Work out the finished part from the listing and answer in its coordinate system (mm). Face numbers are marked on the shaded views. A direction names the side the tool comes from. Coordinates: 2 decimals unless noted, no trailing zeros. Order: outer loops, then holes, each group sorted by start corner. A loop starts at its lowest first (then second) coordinate and runs counter-clockwise, first axis right, second up.
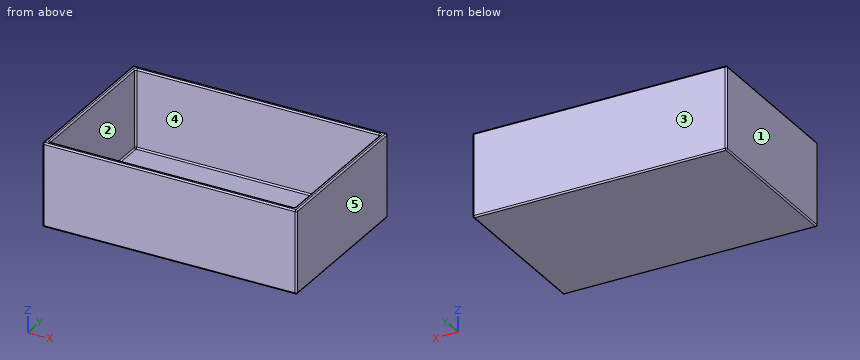
```python
from build123d import *

# Parameters (mm, degrees)
F0_W     = 524.05
F0_H     = 334.05
F0_W_2   = 505
F0_H_2   = 315
F1_DEPTH = 172.025
F2_DEPTH = 9.525
F3_R     = 3


with BuildPart() as f1:
    # F0 (on Top) → F1 (new body)
    with BuildSketch(Plane.XY):
        with Locations((48.210962, 70.14254)):
            Rectangle(F0_W, F0_H)
        with Locations((48.210962, 70.14254)):
            Rectangle(F0_W_2, F0_H_2, mode=Mode.SUBTRACT)
    extrude(amount=F1_DEPTH)

    # F0 (on Top) → F2 (join)
    with BuildSketch(Plane.XY):
        with Locations((48.210962, 70.14254)):
            Rectangle(F0_W_2, F0_H_2)
    extrude(amount=F2_DEPTH)

    # F3
    f3_edges = [f1.edges().sort_by_distance(p)[0] for p in [
        (-213.814038, -96.88246, 86.0125),
        (310.235962, -96.88246, 86.0125),
        (48.210962, -96.88246, 0),
        (48.210962, -96.88246, 172.025),
        (310.235962, 237.16754, 86.0125),
        (310.235962, 70.14254, 0),
        (310.235962, 70.14254, 172.025),
        (-213.814038, 237.16754, 86.0125),
        (48.210962, 237.16754, 0),
        (48.210962, 237.16754, 172.025),
        (-213.814038, 70.14254, 0),
        (-213.814038, 70.14254, 172.025),
        (300.710962, 70.14254, 172.025),
        (48.210962, -87.35746, 172.025),
        (-204.289038, 70.14254, 172.025),
        (48.210962, 227.64254, 172.025),
        (-204.289038, 70.14254, 9.525),
        (-204.289038, 227.64254, 90.775),
        (-204.289038, -87.35746, 90.775),
        (48.210962, -87.35746, 9.525),
        (300.710962, -87.35746, 90.775),
        (300.710962, 70.14254, 9.525),
        (300.710962, 227.64254, 90.775),
        (48.210962, 227.64254, 9.525),
    ]]
    fillet(f3_edges, radius=F3_R)


solid = f1.part
```
1. The part is cut by section C-C (x = -86.5). Determine the outline of the cut face in (y, z) (3 decimals), plus the area to 3 significant figures.
2. The part is cut by section A-A (z = 53.5). Determine the outline of the cut face in (x, y), plus the area to 3 significant figures.
3. For the marked faces 4 and 5, determine the directions among +Z, -Z, +X, -X, +Y, -Y from which every point of the face is accessible in a straight line to the end or side of a thin tool.
4. The part is cut by section B-B (y = 40). Determine the outline of the cut face in (x, z) (3 decimals).
5. The mould has two halves that part along Y. Classify the marked faces 1, 2 and 3: released by +Y, released by -Y, zero draft, split by the parting line, or undercut.
6. A flat-ended cylindrical pin translates along its axis: pin 1 (5 mm diameter, centred on x = -62.5, y = 81, fed in from +Z) (3 decimals). Find the tip coordinate at first contact, or state that the pin passes through.
7. Consider probe 1 along X at (y, z) = (198, 75); probe 2 along Y at (x, z) = (-106, 91); probe 3 along Z at (x, y) = (286.5, 118) (3 decimals). Determine where each line is inside the solid, lowest interval first.
Worked out:
1. outline: (-96.882, 3) arc R3 ccw to (-93.882, 0) - (234.168, 0) arc R3 ccw to (237.168, 3) - (237.168, 169.025) arc R3 ccw to (234.168, 172.025) - (230.643, 172.025) arc R3 ccw to (227.643, 169.025) - (227.643, 12.525) arc R3 cw to (224.643, 9.525) - (-84.357, 9.525) arc R3 cw to (-87.357, 12.525) - (-87.357, 169.025) arc R3 ccw to (-90.357, 172.025) - (-93.882, 172.025) arc R3 ccw to (-96.882, 169.025) - close
1. area: 6,270 mm2
2. outline: (-213.81, -93.88) arc R3 ccw to (-210.81, -96.88) - (307.24, -96.88) arc R3 ccw to (310.24, -93.88) - (310.24, 234.17) arc R3 ccw to (307.24, 237.17) - (-210.81, 237.17) arc R3 ccw to (-213.81, 234.17) - close; hole (-204.29, -84.36) arc R3 ccw to (-201.29, -87.36) - (297.71, -87.36) arc R3 ccw to (300.71, -84.36) - (300.71, 224.64) arc R3 ccw to (297.71, 227.64) - (-201.29, 227.64) arc R3 ccw to (-204.29, 224.64) - close
2. area: 16,000 mm2
3. face 4: +Z
3. face 5: +Z, -Z, +X, +Y, -Y
4. outline: (-213.814, 3) arc R3 ccw to (-210.814, 0) - (307.236, 0) arc R3 ccw to (310.236, 3) - (310.236, 169.025) arc R3 ccw to (307.236, 172.025) - (303.711, 172.025) arc R3 ccw to (300.711, 169.025) - (300.711, 12.525) arc R3 cw to (297.711, 9.525) - (-201.289, 9.525) arc R3 cw to (-204.289, 12.525) - (-204.289, 169.025) arc R3 ccw to (-207.289, 172.025) - (-210.814, 172.025) arc R3 ccw to (-213.814, 169.025) - close
5. face 1: zero draft
5. face 2: undercut
5. face 3: released by +Y
6. pin 1: stops at z = 9.525
7. probe 1: x = -213.81 to -204.29, 300.71 to 310.24
7. probe 2: y = -96.88 to -87.36, 227.64 to 237.17
7. probe 3: z = 0 to 9.525
